from build123d import *

# Parameters (mm, degrees)
SKETCH1_W           = 125
SKETCH1_H           = 125
BOSS_EXTRUDE1_DEPTH = 4
BOSS_EXTRUDE2_DEPTH = 5
SKETCH3_R           = 10
BOSS_EXTRUDE3_DEPTH = 4
SKETCH4_R           = 5.075
CUT_EXTRUDE1_DEPTH  = 4
FILLET1_R           = 125


with BuildPart() as part:
    # Sketch1 → Boss-Extrude1 (new body)
    with BuildSketch(Plane(origin=(0, 0, 0), x_dir=(1, 0, 0), z_dir=(0, 1, 0))):
        Rectangle(SKETCH1_W, SKETCH1_H)
    extrude(amount=BOSS_EXTRUDE1_DEPTH)

    # Sketch2 → Boss-Extrude2 (add)
    with BuildSketch(Plane(origin=(0, 4, 0), x_dir=(1, 0, 0), z_dir=(0, 1, 0))):
        with BuildLine():
            Line((-62.5, -62.5), (-62.5, 62.5))
            Line((-62.5, 62.5), (62.5, 62.5))
            Line((62.5, 62.5), (62.5, 54))
            ThreePointArc((62.5, 54), (-19.877940008, 19.877940008), (-54, -62.5))
            Line((-54, -62.5), (-62.5, -62.5))
        make_face()
    extrude(amount=BOSS_EXTRUDE2_DEPTH)

    # Sketch3 → Boss-Extrude3 (add)
    with BuildSketch(Plane(origin=(0, 4, 0), x_dir=(1, 0, 0), z_dir=(0, 1, 0))):
        with Locations((62.5, -62.5)):
            Circle(SKETCH3_R)
    extrude(amount=-BOSS_EXTRUDE3_DEPTH)

    # Sketch4 → Cut-Extrude1 (cut)
    with BuildSketch(Plane(origin=(0, 4, 0), x_dir=(1, 0, 0), z_dir=(0, 1, 0))):
        with Locations(Location((62.5, -62.5, 0), (0, 0, 270))):
            Circle(SKETCH4_R)
    extrude(amount=-CUT_EXTRUDE1_DEPTH, mode=Mode.SUBTRACT)

    # Fillet1
    fillet1_edges = [part.edges().sort_by_distance(p)[0] for p in [
        (-62.5, 4.5, -62.5),
    ]]
    fillet(fillet1_edges, radius=FILLET1_R - 0.0001)  # a hair under: the kernel refuses the full size


solid = part.part
Can you work these out from the model? Positions are in its coordinate system, mm. A direction names the side the tool comes from. Round coordinates to 2 decimals unless told otherwise and drop trailing zeros. Order: outer loops, then holes, each group sorted by start corner. A loop starts at its lowest first (then second) coordinate and runs counter-clockwise, first axis right, second up. Notation, with made-up numbers: (47.5, 10) - (67.5, 10) arc R5 ccw to (67.5, 17) - close; hole circle Ø10 at (83.25, -34). An arc over 180 degrees is marked (long way). Answer in a Markdown table with one row per item.
(1) Which directions (+Z, -Z, +X, -X, +Y, -Y) give clear straight access to the entire face, cutting with the end or side of a thin tool? Please do faces 5 (the face through (-4, 2, 62.5)), 6 (the face through (69.334, 2.028, 69.8)), 7 (the face through (-18.967, 6.465, -20.779)).
From the geometry:
| item | result |
|---|---|
| face 5 | +Z, -X, +Y, -Y |
| face 6 | +Y, -Y |
| face 7 | +Z, +X, +Y |
(2) For P1, Ø4, axis at x = 42.5, y = 7, coming from the +Z side; P2, Ø1, axis at x = -7, y = 6.5, coming from the -Z side; P3, Ø8, axis at x = 62.5, z = 62.5, coming from the -Y side; P4, Ø1, axis at x = -14.5, y = 6.5, coming from the +Z side, each with a flat end and sliding along its axis, tell me the tip position at first contact or that it passes through.
From the geometry:
| item | result |
|---|---|
| P1 | stops at z = -51.9 |
| P2 | stops at z = -41.73 |
| P3 | passes through |
| P4 | stops at z = -24.48 |
(3) Suppose I cut it at B-B, the plane x = -23.5. Please give me the cut outline in (y, z), plus the area to 3 significant figures.
From the geometry:
| item | result |
|---|---|
| outline | (0, -28.21) - (9, -28.21) - (9, -16.09) - (4, -16.09) - (4, 62.5) - (0, 62.5) - close |
| area | 423 mm2 |
(4) Suppose I cut it at A-A, the plane z = 1.5. Please give me the cut outline in (x, y), plus the area to 3 significant figures.
From the geometry:
| item | result |
|---|---|
| outline | (-46.61, 0) - (62.5, 0) - (62.5, 4) - (-36.75, 4) - (-36.75, 9) - (-46.61, 9) - close |
| area | 486 mm2 |
(5) Please list where these lines run through material, in increasing order: L1, parallel to Y at x = 60, z = 33.5; L2, parallel to Z at x = -3, y = 6.5; L3, parallel to X at y = 5.5, z = -26.5. Write a range as from..to.
From the geometry:
| item | result |
|---|---|
| L1 | y = 0..4 |
| L2 | z = -43.96..-33.84 |
| L3 | x = -25.27..-12.67 |
(6) If we mould it in two halves opening along X, with no side actions, what happens to faces 1 (the face through (67.53, 2.03, 61.84)), 2 (the face through (-26.855, 4.437, -24.911)), 3 (the face through (8, 4, 8)), 4 (the face through (62.5, 2, -6))? For each: released by +X, released by -X, zero draft, split by the parting line, or undercut.
From the geometry:
| item | result |
|---|---|
| face 1 | undercut |
| face 2 | released by -X |
| face 3 | zero draft |
| face 4 | released by +X |
